```python
from build123d import *

# Parameters (mm, degrees)
SKETCH1_R           = 3.175
BOSS_EXTRUDE5_DEPTH = 1.52
SKETCH3_R           = 36
CUT_EXTRUDE4_DEPTH  = 2.52


with BuildPart() as part:
    # Sketch1 → Boss-Extrude5 (new body)
    with BuildSketch(Plane(origin=(0, 0, 0), x_dir=(1, 0, 0), z_dir=(0, 1, 0))):
        with BuildLine():
            Line((-5.999999832, 72.25129758), (-5.999999832, 59.699246243))
            ThreePointArc((-5.999999832, 59.699246243), (-42.426406812, 42.426406931), (-59.699246226, 6))
            Line((-59.699246226, 6), (-72.251297552, 6.000000168))
            ThreePointArc((-72.251297552, 6.000000168), (-72.5, 1.68e-07), (-72.25129758, -5.999999832))
            Line((-72.25129758, -5.999999832), (-59.699246243, -5.999999832))
            ThreePointArc((-59.699246243, -5.999999832), (-42.426406931, -42.426406812), (-6, -59.699246226))
            Line((-6, -59.699246226), (-6.000000168, -72.251297552))
            ThreePointArc((-6.000000168, -72.251297552), (-1.68e-07, -72.5), (5.999999832, -72.25129758))
            Line((5.999999832, -72.25129758), (5.999999832, -59.699246243))
            ThreePointArc((5.999999832, -59.699246243), (42.426406812, -42.426406931), (59.699246226, -6))
            Line((59.699246226, -6), (72.251297552, -6.000000168))
            ThreePointArc((72.251297552, -6.000000168), (72.5, -1.68e-07), (72.25129758, 5.999999832))
            Line((72.25129758, 5.999999832), (59.699246243, 5.999999832))
            ThreePointArc((59.699246243, 5.999999832), (42.426406931, 42.426406812), (6, 59.699246226))
            Line((6, 59.699246226), (6.000000168, 72.251297552))
            ThreePointArc((6.000000168, 72.251297552), (1.68e-07, 72.5), (-5.999999832, 72.25129758))
        make_face()
        with Locations((9.7e-08, 67)):
            Circle(SKETCH1_R, mode=Mode.SUBTRACT)
        with Locations((67, -9.7e-08)):
            Circle(SKETCH1_R, mode=Mode.SUBTRACT)
        with Locations((-9.7e-08, -67)):
            Circle(SKETCH1_R, mode=Mode.SUBTRACT)
        with Locations((-67, 9.7e-08)):
            Circle(SKETCH1_R, mode=Mode.SUBTRACT)
        with BuildLine():
            Line((20.250864517, 30.167050694), (37.571372593, 40.167050694))
            ThreePointArc((37.571372593, 40.167050694), (27.5, 47.631397208), (16, 52.621288468))
            Line((16, 52.621288468), (16, 32.621288468))
            Line((16, 32.621288468), (-16, 32.621288468))
            Line((-16, 32.621288468), (-16, 52.621288468))
            ThreePointArc((-16, 52.621288468), (-27.5, 47.631397208), (-37.571372593, 40.167050694))
            Line((-37.571372593, 40.167050694), (-20.250864517, 30.167050694))
            Line((-20.250864517, 30.167050694), (-36.250864517, 2.454237773))
            Line((-36.250864517, 2.454237773), (-53.571372593, 12.454237773))
            ThreePointArc((-53.571372593, 12.454237773), (-55, 0), (-53.571372593, -12.454237773))
            Line((-53.571372593, -12.454237773), (-36.250864517, -2.454237773))
            Line((-36.250864517, -2.454237773), (-20.250864517, -30.167050694))
            Line((-20.250864517, -30.167050694), (-37.571372593, -40.167050694))
            ThreePointArc((-37.571372593, -40.167050694), (-27.5, -47.631397208), (-16, -52.621288468))
            Line((-16, -52.621288468), (-16, -32.621288468))
            Line((-16, -32.621288468), (16, -32.621288468))
            Line((16, -32.621288468), (16, -52.621288468))
            ThreePointArc((16, -52.621288468), (27.5, -47.631397208), (37.571372593, -40.167050694))
            Line((37.571372593, -40.167050694), (20.250864517, -30.167050694))
            Line((20.250864517, -30.167050694), (36.250864517, -2.454237773))
            Line((36.250864517, -2.454237773), (53.571372593, -12.454237773))
            ThreePointArc((53.571372593, -12.454237773), (55, 0), (53.571372593, 12.454237773))
            Line((53.571372593, 12.454237773), (36.250864517, 2.454237773))
            Line((36.250864517, 2.454237773), (20.250864517, 30.167050694))
        make_face(mode=Mode.SUBTRACT)
    extrude(amount=BOSS_EXTRUDE5_DEPTH)

    # Sketch3 → Cut-Extrude4 (cut, through all)
    with BuildSketch(Plane(origin=(0, 0, 0), x_dir=(1, 0, 0), z_dir=(0, 1, 0))):
        Circle(SKETCH3_R)
    extrude(amount=CUT_EXTRUDE4_DEPTH, mode=Mode.SUBTRACT)


solid = part.part
```
CAD build for the part. Positions are in the model's coordinates, mm. A direction names the side the tool comes from. Round coordinates to 2 decimals unless told otherwise and drop trailing zeros. Order: outer loops, then holes, each group sorted by start corner. A loop starts at its lowest first (then second) coordinate and runs counter-clockwise, first axis right, second up.
Q1. Slice it at D-D (x = -67). Write the cut outline in (y, z) (3 decimals), and give its area (3 significant figures).
Q2. Slice it at A-A (z = 0). Write the cut outline in (x, y) (3 decimals), and give its area (3 significant figures).
Q3. Wall check: L1, parallel to Z at x = -67, y = 0.55 (3 decimals); L2, parallel to X at y = 0.2, z = 50; L3, parallel to Z at x = 25, y = 0.8. Give the ranges that are in metal, low to high.
Q4. Drop flat-ended pins along their axis: pin 1 (5.5 mm diameter, centred on x = 0, z = -67, fed in from +Y); pin 2 (0.5 mm diameter, centred on y = 1, z = 66, fed in from -X); pin 3 (0.9 mm diameter, centred on x = -16, y = 0.5, fed in from -Z); pin 4 (0.5 mm diameter, centred on y = 0.5, z = 47, fed in from +X). Give the stop position or say it passes through.
Q5. Two-plate mould, pull along Z, no slides. Class faces 1 (the cylindrical face through (-42.02, 0.75, -42.83)), 2 (the cylindrical face through (0, 1, 36)), 3 (the cylindrical face through (-42.83, 0.75, 42.02)): pulls with the +Z half, pulls with the -Z half, needs draft (parallel to the pull), parting line crosses it, or undercut.
Q6. Which spindle directions (+Z, -Z, +X, -X, +Y, -Y) get a long thin tool onto all of the face, cutting with end or side? Do faces 4 (the cylindrical face through (-31.066, 0.749, -18.19)), 5 (the flat face through (-33, 0, -16)). Say none if no direction does.
Q7. Slice it at C-C (z = -67). Write the cut outline in (x, y) (3 decimals), and give its area (3 significant figures).
Q8. Slice it at B-B (x = 0). Write the cut outline in (y, z) (3 decimals).
Results below:
1. outline: (0, -6) - (1.52, -6) - (1.52, -3.175) - (0, -3.175) - close; (0, 3.175) - (1.52, 3.175) - (1.52, 6) - (0, 6) - close
1. area: 8.59 mm2
2. outline: (-72.5, 0) - (-70.175, 0) - (-70.175, 1.52) - (-72.5, 1.52) - close; (-63.825, 0) - (-55, 0) - (-55, 1.52) - (-63.825, 1.52) - close; (55, 0) - (63.825, 0) - (63.825, 1.52) - (55, 1.52) - close; (70.175, 0) - (72.5, 0) - (72.5, 1.52) - (70.175, 1.52) - close
2. area: 33.9 mm2
3. L1: z = -6 to -3.175, 3.175 to 6
3. L2: x = -33.17 to -22.91, -16 to 16, 22.91 to 33.17
3. L3: z = -54.54 to -48.99, -32.91 to -25.9, 25.9 to 32.91, 48.99 to 54.54
4. pin 1: passes through
4. pin 2: stops at x = -6
4. pin 3: stops at z = -57.95
4. pin 4: stops at x = 37.61
5. face 1: pulls with the -Z half
5. face 2: undercut
5. face 3: pulls with the +Z half
6. face 4: +Y, -Y
6. face 5: +Z, -Z, +X, -X, -Y
7. outline: (-6, 0) - (-3.175, 0) - (-3.175, 1.52) - (-6, 1.52) - close; (3.175, 0) - (6, 0) - (6, 1.52) - (3.175, 1.52) - close
7. area: 8.59 mm2
8. outline: (0, -72.5) - (1.52, -72.5) - (1.52, -70.175) - (0, -70.175) - close; (0, -63.825) - (1.52, -63.825) - (1.52, -36) - (0, -36) - close; (0, 36) - (1.52, 36) - (1.52, 63.825) - (0, 63.825) - close; (0, 70.175) - (1.52, 70.175) - (1.52, 72.5) - (0, 72.5) - close
